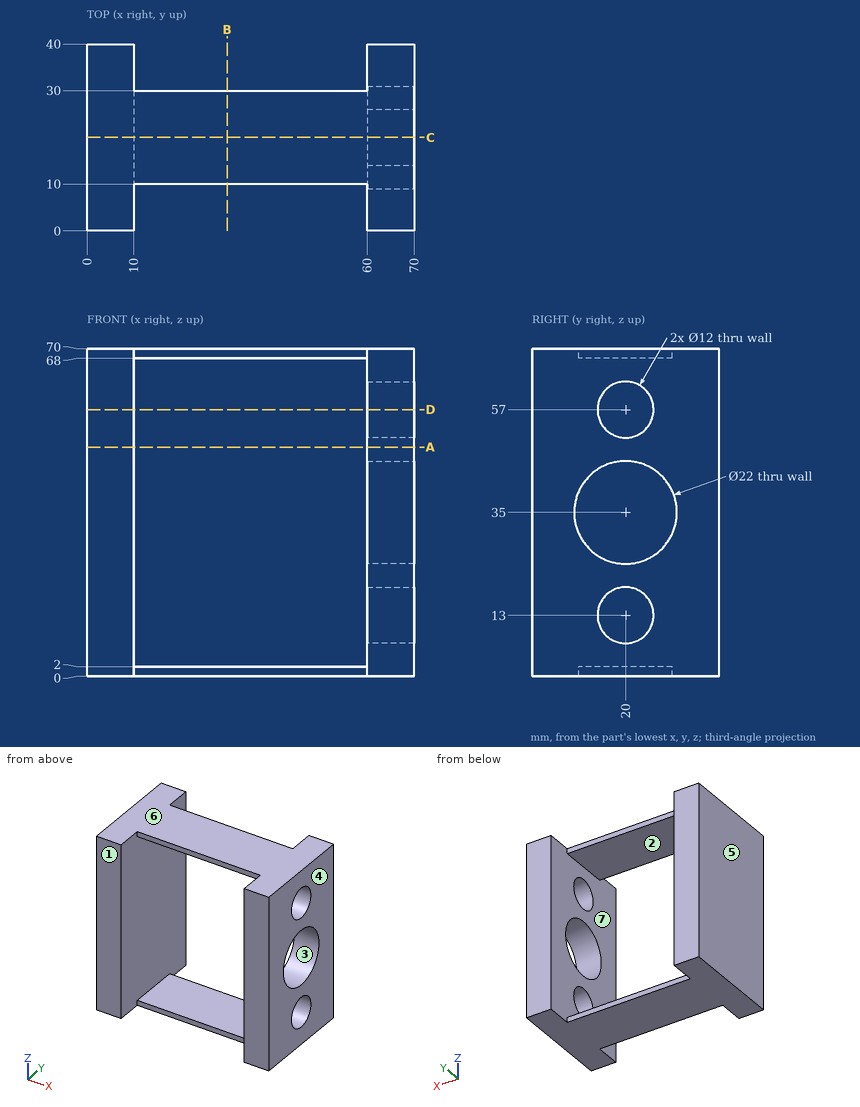
Geometry check sheet. Reference: drawing and pictorial views, mm from the part's lowest x, y, z. A direction names the side the tool comes from. Round coordinates to 2 decimals unless told otherwise and drop trailing zeros. Loops run counter-clockwise (first coordinate to the right, second up) from the corner with the lowest first, then second, coordinate; pieces in that order, holes last. Notation, with made-up numbers: (58, 76.5) -> (104, 76.5) arc R13 ccw to (104, 97.5) -> close; hole circle Ø2 at (-35.75, 18.25). An arc over 180 degrees is marked (long way). Use a Markdown table: item, result.
(1) Sectioned sample at C-C (y = 20). Enter the section's corners in (x, z), then the cut area to 3 significant figures.
Calculated:
| item | result |
|---|---|
| outline | (0, 0) -> (70, 0) -> (70, 7) -> (60, 7) -> (60, 2) -> (10, 2) -> (10, 68) -> (60, 68) -> (60, 63) -> (70, 63) -> (70, 70) -> (0, 70) -> close; (60, 19) -> (70, 19) -> (70, 24) -> (60, 24) -> close; (60, 46) -> (70, 46) -> (70, 51) -> (60, 51) -> close |
| area | 1,140 mm² |
(2) Sectioned sample at A-A (z = 49). Enter the section's corners in (x, y).
Calculated:
| item | result |
|---|---|
| outline | (0, 0) -> (10, 0) -> (10, 40) -> (0, 40) -> close; (60, 0) -> (70, 0) -> (70, 40) -> (60, 40) -> close |
(3) Scan lines: probe 1 along X at (y, z) = (35, 17.5); probe 2 along Z at (x, y) = (51, 18); probe 3 along Y at (x, z) = (66, 13). Record each from-to range of solid material in increasing order.
Calculated:
| item | result |
|---|---|
| probe 1 | 0 to 10, 60 to 70 |
| probe 2 | 0 to 2, 68 to 70 |
| probe 3 | 0 to 14, 26 to 40 |
(4) Sectioned sample at B-B (x = 30). Enter the section's corners in (y, z), then the cut area to 3 significant figures.
Calculated:
| item | result |
|---|---|
| outline | (10, 0) -> (30, 0) -> (30, 2) -> (10, 2) -> close; (10, 68) -> (30, 68) -> (30, 70) -> (10, 70) -> close |
| area | 80.0 mm² |
(5) Set-up check for the marked faces 1, 2 and 3: record each of +Z, -Z, +X, -X, +Y, -Y from which the full face is reachable in a straight line by a thin tool's end or side.
Calculated:
| item | result |
|---|---|
| face 1 | +Z, -Z, +X, -X, -Y |
| face 2 | +Y, -Y |
| face 3 | +X |
(6) Go/stop test with flat-tipped pins: P1, Ø7, axis at y = 20, z = 57, coming from the +X side; P2, Ø0.6, axis at x = 30.5, z = 1.5, coming from the -Y side; P3, Ø2, axis at x = 37, z = 69.5, coming from the +Y side. Record where each tip stops, or that it passes through.
Calculated:
| item | result |
|---|---|
| P1 | x = 10 |
| P2 | y = 10 |
| P3 | y = 30 |
(7) Sectioned sample at D-D (z = 57). Enter the section's corners in (x, y), then the cut area to 3 significant figures.
Calculated:
| item | result |
|---|---|
| outline | (0, 0) -> (10, 0) -> (10, 40) -> (0, 40) -> close; (60, 0) -> (70, 0) -> (70, 14) -> (60, 14) -> close; (60, 26) -> (70, 26) -> (70, 40) -> (60, 40) -> close |
| area | 680 mm² |
(8) Mould release check, pull along X, two halves, no side actions. Record for the marked faces 4, 5, 6 and 7: released by +X, released by -X, zero draft, split by the parting line, or undercut.
Calculated:
| item | result |
|---|---|
| face 4 | released by +X |
| face 5 | released by -X |
| face 6 | zero draft |
| face 7 | undercut |
